from build123d import *

# Parameters (mm, degrees)
F0_W          = 102.1880283952
F0_H          = 23.8108858466
F1_DEPTH      = 38.1
F2_R          = 11.9054429233
F3_DEPTH      = 63.5
F4_W          = 86.9480283952
F4_H          = 88.2315921943
F5_DEPTH      = 25.4
F6_R          = 2.54
F7_DEPTH      = 63.5
F8_T1_DEPTH   = 127.5880283952
F8_T6_DEPTH   = 101.6
F8_S7_R       = 11.9054429233
F8_T8_DEPTH   = 52
F8_T12_DEPTH  = 101.6
F8_S13_R      = 11.9054429233
F8_T14_DEPTH  = 52
F9_T1_DEPTH   = 127.5880283952
F9_T6_DEPTH   = 101.6
F9_S7_R       = 11.9054429233
F9_T8_DEPTH   = 52
F9_T12_DEPTH  = 101.6
F9_S13_R      = 11.9054429233
F9_T14_DEPTH  = 52
F10_T1_DEPTH  = 13.6508858466
F10_S5_W      = 5.08
F10_S5_H      = 5.08
F10_T6_DEPTH  = 5.08
F10_S11_W     = 5.08
F10_S11_H     = 5.08
F10_T12_DEPTH = 5.08
F10_S17_W     = 5.08
F10_S17_H     = 5.08
F10_T18_DEPTH = 5.08
F10_S23_W     = 5.08
F10_S23_H     = 5.08
F10_T24_DEPTH = 5.08
F11_R         = 5.08
F12_R         = 2.53999


# Not quite as in the source:
# - a fillet or chamfer that OpenCascade refuses, or shapes differently, is made with other operations: its cross-section is extruded or revolved along the edge and cut away or added
# - a fillet or chamfer is up to 0.001 mm smaller than in the source, because OpenCascade refuses the exact size


with BuildPart() as f1:
    # F0 (on Top) → F1 (new body, symmetric)
    with BuildSketch(Plane.XY):
        Rectangle(F0_W, F0_H)
    extrude(amount=F1_DEPTH, both=True)

    # F2 (on Right) → F3 (join, symmetric)
    with BuildSketch(Plane.YZ):
        with Locations((0, 38.1)):
            Circle(F2_R)
    extrude(amount=F3_DEPTH, both=True)

    # F4 (on Front) → F5 (cut, symmetric)
    with BuildSketch(Plane.XZ):
        with Locations((0, 18.7157960971)):
            Rectangle(F4_W, F4_H)
    extrude(amount=F5_DEPTH, both=True, mode=Mode.SUBTRACT)

    # F6 (on Right) → F7 (cut, symmetric)
    with BuildSketch(Plane.YZ):
        with Locations((0, 38.1)):
            Circle(F6_R)
    extrude(amount=F7_DEPTH, both=True, mode=Mode.SUBTRACT)

    # F8: fillet of radius 5.08 on 3 edges, made by hand

    # F8_s2 → F8_t1 (cut)
    with BuildSketch(Plane.YZ.offset(-63.7940141976)):
        with BuildLine():
            ThreePointArc((-6.8254429233, -38.1), (-10.4175453717, -36.6121024484), (-11.9054429233, -33.02))
            Line((-11.9054429233, -33.02), (-11.9054429233, -38.1))
            Line((-11.9054429233, -38.1), (-6.8254429233, -38.1))
        make_face()
    extrude(amount=F8_T1_DEPTH, mode=Mode.SUBTRACT)


with BuildPart() as f8_tool4:
    # F8_s5 → F8_t6 (new body)
    with BuildSketch(Plane.XY.offset(50.8)):
        with BuildLine():
            ThreePointArc((51.0940141976, -6.8254429233), (49.606116646, -10.4175453717), (46.0140141976, -11.9054429233))
            Line((46.0140141976, -11.9054429233), (51.0940141976, -11.9054429233))
            Line((51.0940141976, -11.9054429233), (51.0940141976, -6.8254429233))
        make_face()
    extrude(amount=-F8_T6_DEPTH)

    # F8_s7 → F8_t8 (cut, symmetric)
    with BuildSketch(Plane.YZ.offset(48.6)):
        with Locations((0, 38.1)):
            Circle(F8_S7_R)
    extrude(amount=F8_T8_DEPTH, both=True, mode=Mode.SUBTRACT)


with BuildPart() as f1_1:
    add(f1.part)

    # F8_t3: cut F8_tool4
    add(f8_tool4.part, mode=Mode.SUBTRACT)


with BuildPart() as f8_tool10:
    # F8_s11 → F8_t12 (new body)
    with BuildSketch(Plane.XY.offset(-50.8)):
        with BuildLine():
            ThreePointArc((-51.0940141976, -6.8254429233), (-49.606116646, -10.4175453717), (-46.0140141976, -11.9054429233))
            Line((-46.0140141976, -11.9054429233), (-51.0940141976, -11.9054429233))
            Line((-51.0940141976, -11.9054429233), (-51.0940141976, -6.8254429233))
        make_face()
    extrude(amount=F8_T12_DEPTH)

    # F8_s13 → F8_t14 (cut, symmetric)
    with BuildSketch(Plane.YZ.offset(-48.6)):
        with Locations((0, 38.1)):
            Circle(F8_S13_R)
    extrude(amount=F8_T14_DEPTH, both=True, mode=Mode.SUBTRACT)


with BuildPart() as f1_2:
    add(f1_1.part)

    # F8_t9: cut F8_tool10
    add(f8_tool10.part, mode=Mode.SUBTRACT)

    # F9: fillet of radius 5.08 on 3 edges, made by hand

    # F9_s2 → F9_t1 (cut)
    with BuildSketch(Plane.YZ.offset(-63.7940141976)):
        with BuildLine():
            ThreePointArc((11.9054429233, -33.02), (10.4175453717, -36.6121024484), (6.8254429233, -38.1))
            Line((6.8254429233, -38.1), (11.9054429233, -38.1))
            Line((11.9054429233, -38.1), (11.9054429233, -33.02))
        make_face()
    extrude(amount=F9_T1_DEPTH, mode=Mode.SUBTRACT)


with BuildPart() as f9_tool4:
    # F9_s5 → F9_t6 (new body)
    with BuildSketch(Plane.XY.offset(-50.8)):
        with BuildLine():
            ThreePointArc((-46.0140141976, 11.9054429233), (-49.606116646, 10.4175453717), (-51.0940141976, 6.8254429233))
            Line((-51.0940141976, 6.8254429233), (-51.0940141976, 11.9054429233))
            Line((-51.0940141976, 11.9054429233), (-46.0140141976, 11.9054429233))
        make_face()
    extrude(amount=F9_T6_DEPTH)

    # F9_s7 → F9_t8 (cut, symmetric)
    with BuildSketch(Plane.YZ.offset(-48.6)):
        with Locations((0, 38.1)):
            Circle(F9_S7_R)
    extrude(amount=F9_T8_DEPTH, both=True, mode=Mode.SUBTRACT)


with BuildPart() as f1_3:
    add(f1_2.part)

    # F9_t3: cut F9_tool4
    add(f9_tool4.part, mode=Mode.SUBTRACT)


with BuildPart() as f9_tool10:
    # F9_s11 → F9_t12 (new body)
    with BuildSketch(Plane.XY.offset(50.8)):
        with BuildLine():
            ThreePointArc((46.0140141976, 11.9054429233), (49.606116646, 10.4175453717), (51.0940141976, 6.8254429233))
            Line((51.0940141976, 6.8254429233), (51.0940141976, 11.9054429233))
            Line((51.0940141976, 11.9054429233), (46.0140141976, 11.9054429233))
        make_face()
    extrude(amount=-F9_T12_DEPTH)

    # F9_s13 → F9_t14 (cut, symmetric)
    with BuildSketch(Plane.YZ.offset(48.6)):
        with Locations((0, 38.1)):
            Circle(F9_S13_R)
    extrude(amount=F9_T14_DEPTH, both=True, mode=Mode.SUBTRACT)


with BuildPart() as f1_4:
    add(f1_3.part)

    # F9_t9: cut F9_tool10
    add(f9_tool10.part, mode=Mode.SUBTRACT)

    # F10: fillet of radius 5.08 on 2 edges, made by hand

    # F10_s2 → F10_t1 (cut)
    with BuildSketch(Plane.XZ.offset(-6.8254429233)):
        with BuildLine():
            ThreePointArc((-46.0140141976, -38.1), (-49.606116646, -36.6121024484), (-51.0940141976, -33.02))
            Line((-51.0940141976, -33.02), (-51.0940141976, -38.1))
            Line((-51.0940141976, -38.1), (-46.0140141976, -38.1))
        make_face()
        with BuildLine():
            ThreePointArc((46.0140141976, -38.1), (49.606116646, -36.6121024484), (51.0940141976, -33.02))
            Line((51.0940141976, -33.02), (51.0940141976, -38.1))
            Line((51.0940141976, -38.1), (46.0140141976, -38.1))
        make_face()
    extrude(amount=F10_T1_DEPTH, mode=Mode.SUBTRACT)


with BuildPart() as f10_tool4:
    # F10_s5 → F10_t6 (new body)
    with BuildSketch(Plane.XY.offset(-33.02)):
        with Locations((48.5540141976, -9.3654429233)):
            Rectangle(F10_S5_W, F10_S5_H)
    extrude(amount=-F10_T6_DEPTH)

    # F10_s7 → F10_t8 (revolve, cut)
    with BuildSketch(Plane(origin=(46.0140141976, -6.8254429233, -33.02), x_dir=(-0.7071067812, 0.7071067812, 0), z_dir=(-0.7071067812, -0.7071067812, 0))):
        with BuildLine():
            ThreePointArc((0, -5.08), (5.08, 0), (0, 5.08))
            Line((0, 5.08), (0, -5.08))
        make_face()
    revolve(axis=Axis((46.0140141976, -6.8254429233, -33.02), (0, 0, -1)), mode=Mode.SUBTRACT)


with BuildPart() as f1_5:
    add(f1_4.part)

    # F10_t3: cut F10_tool4
    add(f10_tool4.part, mode=Mode.SUBTRACT)


with BuildPart() as f10_tool10:
    # F10_s11 → F10_t12 (new body)
    with BuildSketch(Plane.XY.offset(-33.02)):
        with Locations((48.5540141976, 9.3654429233)):
            Rectangle(F10_S11_W, F10_S11_H)
    extrude(amount=-F10_T12_DEPTH)

    # F10_s13 → F10_t14 (revolve, cut)
    with BuildSketch(Plane(origin=(46.0140141976, 6.8254429233, -33.02), x_dir=(-0.7071067812, -0.7071067812, 0), z_dir=(0.7071067812, -0.7071067812, 0))):
        with BuildLine():
            ThreePointArc((0, -5.08), (5.08, 0), (0, 5.08))
            Line((0, 5.08), (0, -5.08))
        make_face()
    revolve(axis=Axis((46.0140141976, 6.8254429233, -33.02), (0, 0, -1)), mode=Mode.SUBTRACT)


with BuildPart() as f1_6:
    add(f1_5.part)

    # F10_t9: cut F10_tool10
    add(f10_tool10.part, mode=Mode.SUBTRACT)


with BuildPart() as f10_tool16:
    # F10_s17 → F10_t18 (new body)
    with BuildSketch(Plane.XY.offset(-33.02)):
        with Locations((-48.5540141976, 9.3654429233)):
            Rectangle(F10_S17_W, F10_S17_H)
    extrude(amount=-F10_T18_DEPTH)

    # F10_s19 → F10_t20 (revolve, cut)
    with BuildSketch(Plane(origin=(-46.0140141976, 6.8254429233, -33.02), x_dir=(0.7071067812, -0.7071067812, 0), z_dir=(0.7071067812, 0.7071067812, 0))):
        with BuildLine():
            ThreePointArc((0, -5.08), (5.08, 0), (0, 5.08))
            Line((0, 5.08), (0, -5.08))
        make_face()
    revolve(axis=Axis((-46.0140141976, 6.8254429233, -33.02), (0, 0, -1)), mode=Mode.SUBTRACT)


with BuildPart() as f1_7:
    add(f1_6.part)

    # F10_t15: cut F10_tool16
    add(f10_tool16.part, mode=Mode.SUBTRACT)


with BuildPart() as f10_tool22:
    # F10_s23 → F10_t24 (new body)
    with BuildSketch(Plane.XY.offset(-33.02)):
        with Locations((-48.5540141976, -9.3654429233)):
            Rectangle(F10_S23_W, F10_S23_H)
    extrude(amount=-F10_T24_DEPTH)

    # F10_s25 → F10_t26 (revolve, cut)
    with BuildSketch(Plane(origin=(-46.0140141976, -6.8254429233, -33.02), x_dir=(0.7071067812, 0.7071067812, 0), z_dir=(-0.7071067812, 0.7071067812, 0))):
        with BuildLine():
            ThreePointArc((0, -5.08), (5.08, 0), (0, 5.08))
            Line((0, 5.08), (0, -5.08))
        make_face()
    revolve(axis=Axis((-46.0140141976, -6.8254429233, -33.02), (0, 0, -1)), mode=Mode.SUBTRACT)


with BuildPart() as f1_8:
    add(f1_7.part)

    # F10_t21: cut F10_tool22
    add(f10_tool22.part, mode=Mode.SUBTRACT)

    # F11
    f11_edges = [f1_8.edges().sort_by_distance(p)[0] for p in [
        (-43.474014, 0, -25.4),
        (43.474014, 0, -25.4),
    ]]
    fillet(f11_edges, radius=F11_R)

    # F12 (radius 2.54 in the source; OpenCascade refuses exactly that, so slightly less here)
    f12_edges = [f1_8.edges().sort_by_distance(p)[0] for p in [
        (0, -11.905443, -25.4),
        (-43.474014, -11.905443, 8.89),
        (-41.986117, -11.905443, -23.912102),
        (41.986117, -11.905443, -23.912102),
        (43.474014, -11.905443, 8.89),
    ]]
    fillet(f12_edges, radius=F12_R)


solid = f1_8.part
Geometry: final body of the model. Coordinates: model frame, mm. A direction names the side the tool comes from. Coordinates: 2 decimals unless noted, no trailing zeros. Order: outer loops, then holes, each group sorted by start corner. A loop starts at its lowest first (then second) coordinate and runs counter-clockwise, first axis right, second up.
(1) Access query for faces 1 (the face through (41.95, -0.13, -23.95)), 2 (the face through (49.566, 10.457, 3.038)), 3 (the face through (-54.635, -1.55, 49.904)), 4 (the face through (-44.238, -11.181, 8.481)). Directions: +Z, -Z, +X, -X, +Y, -Y. A direction counts if a zero-diameter tool reaches every point of the face in a straight line with its end or side. Return the directions, or none.
(2) Draft query along X for faces 5 (the face through (51.094, 0, -2)), 6 (the face through (0, -11.905, -29)), 7 (the face through (-49.645, -10.378, 2.042)), 8 (the face through (-44.238, 11.181, 9.299)). Return one class per face: pulls with the +X half, pulls with the -X half, needs draft (parallel to the pull), parting line crosses it, or undercut.
(3) Material intervals for probe 1 along X at (y, z) = (7, 44); probe 2 along Z at (x, y) = (55.75, 0); probe 3 along X at (y, z) = (5.75, 7), sorted ascending.
(4) Section query C-C (x = -47.5). Return the cut outline in (y, z).
(5) First-contact query: pin 1 (8 mm diameter, centred on y = -8, z = -8, fed in from +X); pin 2 (5 mm diameter, centred on x = 22, y = 7.5, fed in from +Z); pin 3 (4.5 mm diameter, centred on y = 0, z = 38.1, fed in from +X); pin 4 (2 mm diameter, centred on x = -7.5, y = -9, fed in from -Z). Flat tips, straight axial feed; report the tip coordinate or a pass-through.
(6) Section query B-B (y = 0). Return the cut outline in (x, z).
(7) Section query D-D (x = 34.5). Return the cut outline in (y, z).
Solution:
1. face 1: +Z, +Y, -Y
1. face 2: -Z, +X, +Y
1. face 3: -X
1. face 4: +Z, -Y
2. face 5: pulls with the +X half
2. face 6: needs draft
2. face 7: pulls with the -X half
2. face 8: undercut
3. probe 1: x = -63.5 to -43.47, 43.47 to 63.5
3. probe 2: z = 26.19 to 35.56, 40.64 to 50.01
3. probe 3: x = -51.09 to -43.47, 43.47 to 51.09
4. outline: (-11.68, -33.02) arc R4.86 ccw to (-6.83, -37.88) - (6.83, -37.88) arc R4.86 ccw to (11.68, -33.02) - (11.68, 35.81) arc R11.91 ccw (long way) to (-11.68, 35.81) - close; hole circle Ø5.08 at (0, 38.1)
5. pin 1: stops at x = 51.09
5. pin 2: stops at z = -25.4
5. pin 3: passes through
5. pin 4: stops at z = -37.96
6. outline: (-63.5, 26.19) - (-51.09, 26.19) - (-51.09, -33.02) arc R5.08 ccw to (-46.01, -38.1) - (46.01, -38.1) arc R5.08 ccw to (51.09, -33.02) - (51.09, 26.19) - (63.5, 26.19) - (63.5, 35.56) - (43.47, 35.56) - (43.47, -20.32) arc R5.08 cw to (38.39, -25.4) - (-38.39, -25.4) arc R5.08 cw to (-43.47, -20.32) - (-43.47, 35.56) - (-63.5, 35.56) - close; (-63.5, 40.64) - (-43.47, 40.64) - (-43.47, 47.47) arc R2.54 ccw to (-46.01, 50.01) - (-63.5, 50.01) - close; (43.47, 40.64) - (63.5, 40.64) - (63.5, 50.01) - (46.01, 50.01) arc R2.54 ccw to (43.47, 47.47) - close
7. outline: (-11.91, -33.02) arc R5.08 ccw to (-6.83, -38.1) - (6.83, -38.1) arc R5.08 ccw to (11.91, -33.02) - (11.91, -27.94) arc R2.54 ccw to (9.37, -25.4) - (-9.37, -25.4) arc R2.54 ccw to (-11.91, -27.94) - close
